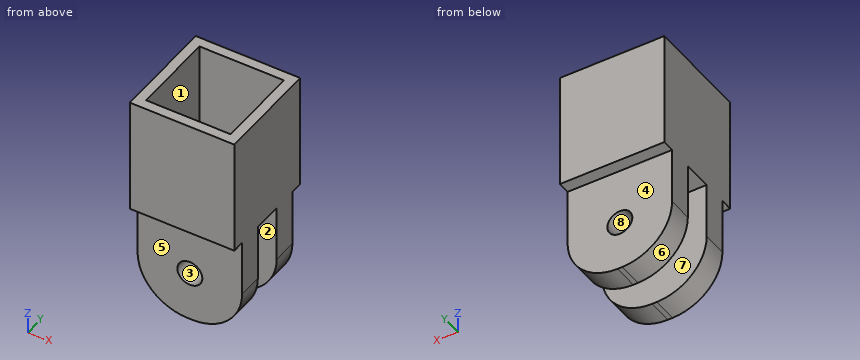
from build123d import *

# Parameters (mm, degrees)
SKETCH1_W           = 31.4
SKETCH1_H           = 31.4
SKETCH1_W_2         = 25.4
SKETCH1_H_2         = 25.4
BOSS_EXTRUDE1_DEPTH = 30
SKETCH2_W           = 31.4
SKETCH2_H           = 31.4
BOSS_EXTRUDE2_DEPTH = 5
SKETCH3_W           = 31.4
SKETCH3_H           = 7.5
BOSS_EXTRUDE3_DEPTH = 5
SKETCH6_R           = 3.75
BOSS_EXTRUDE6_DEPTH = 7.5


with BuildPart() as part:
    # Sketch1 → Boss-Extrude1 (new body)
    with BuildSketch(Plane.XY):
        Rectangle(SKETCH1_W, SKETCH1_H)
        Rectangle(SKETCH1_W_2, SKETCH1_H_2, mode=Mode.SUBTRACT)
    extrude(amount=BOSS_EXTRUDE1_DEPTH)

    # Sketch2 → Boss-Extrude2 (add)
    with BuildSketch(Plane(origin=(0, 0, 0), x_dir=(-1, 0, 0), z_dir=(0, 0, -1))):
        Rectangle(SKETCH2_W, SKETCH2_H)
    extrude(amount=BOSS_EXTRUDE2_DEPTH)

    # Sketch3 → Boss-Extrude3 (add)
    with BuildSketch(Plane(origin=(0, 0, -5), x_dir=(-1, 0, 0), z_dir=(0, 0, -1))):
        with Locations((0, 8.25)):
            Rectangle(SKETCH3_W, SKETCH3_H)
    boss_extrude3 = extrude(amount=BOSS_EXTRUDE3_DEPTH)

    # Sketch6 → Boss-Extrude6 (add)
    with BuildSketch(Plane(origin=(0, 12, 0), x_dir=(1, 0, 0), z_dir=(0, 1, 0))):
        with BuildLine():
            Line((-15.7, 10), (-15.7, 22))
            ThreePointArc((-15.7, 22), (-11.306601718, 32.606601718), (-0.7, 37))
            Line((-0.7, 37), (0.7, 37))
            ThreePointArc((0.7, 37), (11.306601718, 32.606601718), (15.7, 22))
            Line((15.7, 22), (15.7, 10))
            Line((15.7, 10), (-15.7, 10))
        make_face()
        with Locations(Location((0, 22, 0), (0, 0, 270))):
            Circle(SKETCH6_R, mode=Mode.SUBTRACT)
    boss_extrude6 = extrude(amount=-BOSS_EXTRUDE6_DEPTH)

    # Mirror1: Boss-Extrude3, Boss-Extrude6 across plane
    add(boss_extrude3.mirror(Plane.ZX))
    add(boss_extrude6.mirror(Plane.ZX))


solid = part.part
Work out the finished part from the listing and answer in its coordinate system (mm). Face numbers are marked on the shaded views. A direction names the side the tool comes from. Round coordinates to 2 decimals unless told otherwise and drop trailing zeros. Loops run counter-clockwise (first coordinate to the right, second up) from the corner with the lowest first, then second, coordinate; pieces in that order, holes last. Notation, with made-up numbers: (61, 67.25) - (83, 67.25) arc R22 cw to (83, 76.25) - close; hole circle Ø7 at (12.25, -35.5). An arc over 180 degrees is marked (long way). Use one line per item in the form item = value. Start each with the question number.
(1) Flat-ended cylindrical pins translate along their axes: P1, Ø1.1, axis at x = 5.5, y = 14.5, coming from the -Z side; P2, Ø15.5, axis at x = -1.5, z = -26, coming from the +Y side; P3, Ø6, axis at x = 0, z = -22, coming from the +Y side; P4, Ø4, axis at x = 6, y = -13.5, coming from the -Z side. Find the tip coordinate at first contact, or state that the pin passes through.
(2) Find section B-B on y = -8. Determine the outline of the cut face in (x, z).
(3) Find section C-C on z = -24.5. Determine the outline of the cut face in (x, y), and give its area (3 significant figures).
(4) Find section D-D on z = -10. Determine the outline of the cut face in (x, y).
(5) Find section A-A on x = 0. Determine the outline of the cut face in (y, z), and give its area (4 significant figures).
(6) Consider line 1 (X direction, y = -2, z = 11.5); line 2 (Y direction, x = -1, z = -14.5); line 3 (X direction, y = -9, z = -22). Determine where each line is inside the solid, lowest interval first.
(7) Which of the six approach directions +Z, -Z, +X, -X, +Y, -Y give full straight-line access (tool end or side, diameter ignored) to the marked faces 1, 2, 3, 4 and 5?
(8) Determine the mould class of the marked faces 6, 7 and 8 for opening direction Z: +Z half, -Z half, draft (parallel to the pull), parting line (faces both ways), or undercut.
Answer list:
q1.P1 = -5
q1.P2 = 12
q1.P3 = through
q1.P4 = -36.46
q2.outline = (-15.7, -22) arc R15 ccw to (-0.7, -37) - (0.7, -37) arc R15 ccw to (15.7, -22) - (15.7, 30) - (12.7, 30) - (12.7, 0) - (-12.7, 0) - (-12.7, 30) - (-15.7, 30) - close; hole circle Ø7.5 at (0, -22)
q3.outline = (-15.49, -12) - (-2.8, -12) - (-2.8, -4.5) - (-15.49, -4.5) - close; (-15.49, 4.5) - (-2.8, 4.5) - (-2.8, 12) - (-15.49, 12) - close; (2.8, -12) - (15.49, -12) - (15.49, -4.5) - (2.8, -4.5) - close; (2.8, 4.5) - (15.49, 4.5) - (15.49, 12) - (2.8, 12) - close
q3.area = 381 mm^2
q4.outline = (-15.7, -12) - (15.7, -12) - (15.7, -4.5) - (-15.7, -4.5) - close; (-15.7, 4.5) - (15.7, 4.5) - (15.7, 12) - (-15.7, 12) - close
q5.outline = (-15.7, -5) - (-12, -5) - (-12, -18.25) - (-4.5, -18.25) - (-4.5, -5) - (4.5, -5) - (4.5, -18.25) - (12, -18.25) - (12, -5) - (15.7, -5) - (15.7, 30) - (12.7, 30) - (12.7, 0) - (-12.7, 0) - (-12.7, 30) - (-15.7, 30) - close; (-12, -37) - (-4.5, -37) - (-4.5, -25.75) - (-12, -25.75) - close; (4.5, -37) - (12, -37) - (12, -25.75) - (4.5, -25.75) - close
q5.area = 704.5 mm^2
q6.line_1 = -15.7 to -12.7, 12.7 to 15.7
q6.line_2 = -12 to -4.5, 4.5 to 12
q6.line_3 = -15.7 to -3.75, 3.75 to 15.7
q7.face_1 = +Z
q7.face_2 = -Z, +X, -X
q7.face_3 = +Y, -Y
q7.face_4 = -Z, +X, -X, +Y
q7.face_5 = -Z, +X, -X, -Y
q8.face_6 = -Z half
q8.face_7 = draft
q8.face_8 = undercut
